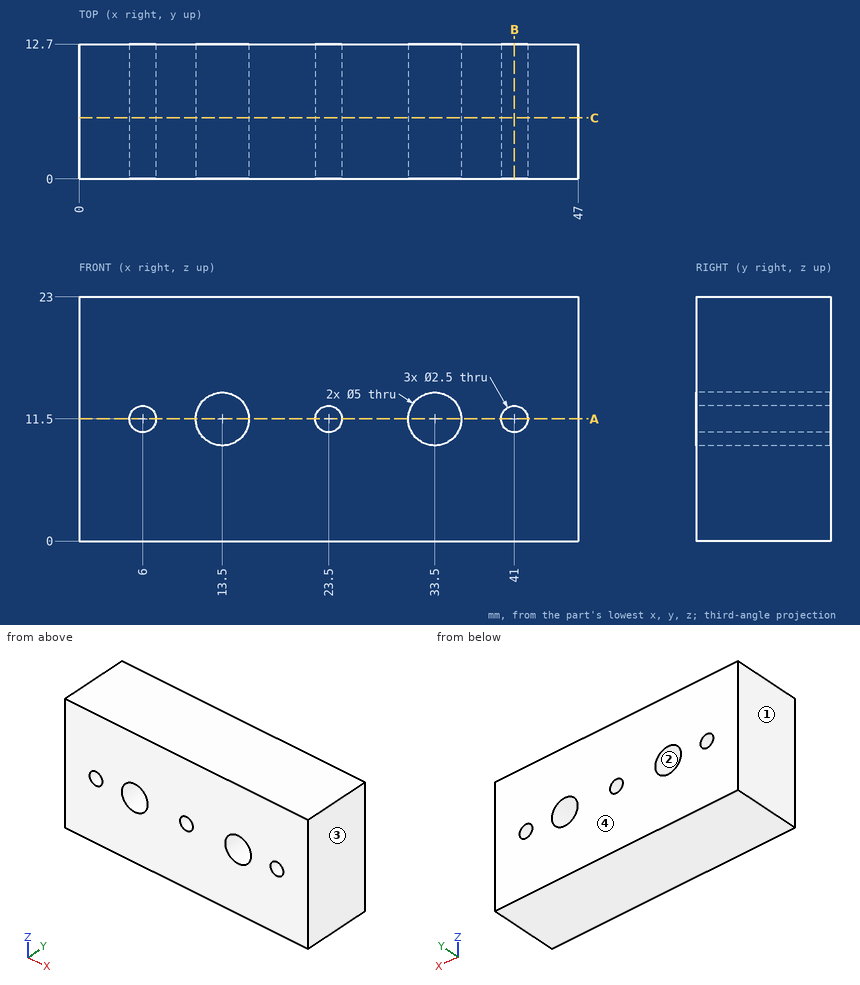
Source: three-view drawing plus pictorial views. Frame: mm from the lowest corner of the part. Round coordinates to 2 decimals unless told otherwise and drop trailing zeros. Loops run counter-clockwise (first coordinate to the right, second up) from the corner with the lowest first, then second, coordinate; pieces in that order, holes last.
Item 1: Mould query, pull axis X, two halves, no side actions, for the marked faces 1, 2, 3 and 4. Classes: released by +X, released by -X, zero draft, split by the parting line, or undercut.
Checked values:
face 1: released by -X
face 2: undercut
face 3: released by +X
face 4: zero draft
Item 2: Section C-C, the plane y = 5.75. Output: boundary loops of the cut face in (x, z).
Checked values:
outline: (0, 0) - (47, 0) - (47, 23) - (0, 23) - close; hole circle Ø2.5 at (6, 11.5); hole circle Ø5 at (13.5, 11.5); hole circle Ø2.5 at (23.5, 11.5); hole circle Ø5 at (33.5, 11.5); hole circle Ø2.5 at (41, 11.5)
Item 3: Contact query for flat-ended pins moving along their axis: P1, Ø1.5, axis at x = 34.5, z = 14, coming from the -Y side; P2, Ø4, axis at x = 33.5, z = 11.5, coming from the -Y side. Output: stop coordinate, or through.
Checked values:
P1: stops at y = 0
P2: passes through
Item 4: Section B-B, the plane x = 41. Output: boundary loops of the cut face in (y, z).
Checked values:
outline: (0, 0) - (12.7, 0) - (12.7, 10.25) - (0, 10.25) - close; (0, 12.75) - (12.7, 12.75) - (12.7, 23) - (0, 23) - close
Item 5: Line query: L1, parallel to X at y = 4, z = 11.5; L2, parallel to X at y = 1, z = 9.75; L3, parallel to Z at x = 41, y = 7. Output: solid intervals per line, ascending.
Checked values:
L1: x = 0 to 4.75, 7.25 to 11, 16 to 22.25, 24.75 to 31, 36 to 39.75, 42.25 to 47
L2: x = 0 to 11.71, 15.29 to 31.71, 35.29 to 47
L3: z = 0 to 10.25, 12.75 to 23
Item 6: Section A-A, the plane z = 11.5. Output: boundary loops of the cut face in (x, y), plus the area to 3 significant figures.
Checked values:
outline: (0, 0) - (4.75, 0) - (4.75, 12.7) - (0, 12.7) - close; (7.25, 0) - (11, 0) - (11, 12.7) - (7.25, 12.7) - close; (16, 0) - (22.25, 0) - (22.25, 12.7) - (16, 12.7) - close; (24.75, 0) - (31, 0) - (31, 12.7) - (24.75, 12.7) - close; (36, 0) - (39.75, 0) - (39.75, 12.7) - (36, 12.7) - close; (42.25, 0) - (47, 0) - (47, 12.7) - (42.25, 12.7) - close
area: 375 mm2
